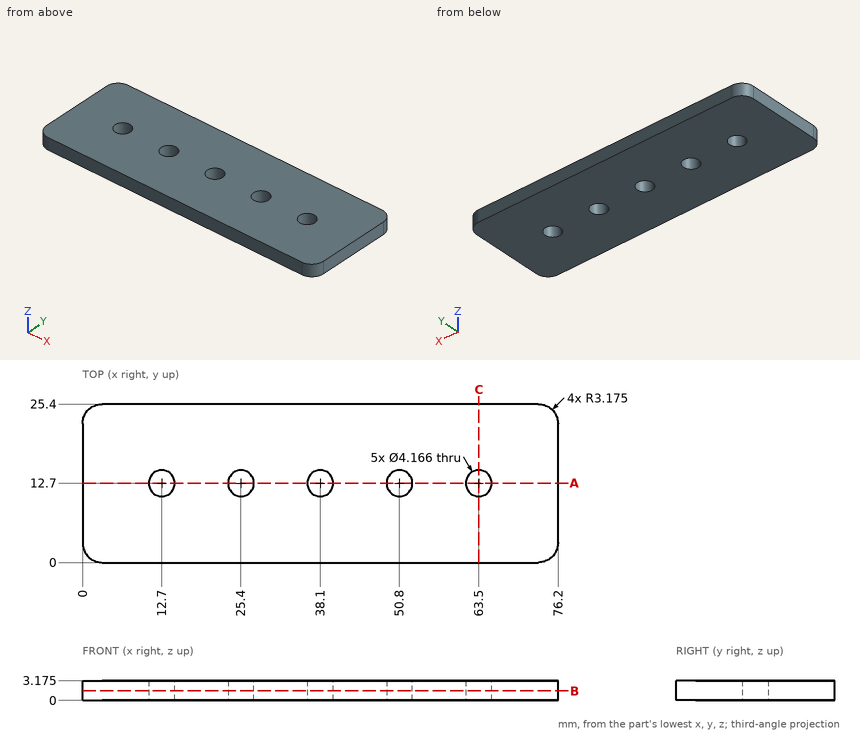
Job drawing, mm, ordinate dimensions from the low corner. One solid piece. Give positions to 0.01 mm unless a question says otherwise; leave off trailing zeros. Write each loop counter-clockwise with the first axis right and the second up, starting at its lowest first coordinate (ties: lowest second). Pieces come first, ordered by that corner, then holes. Notation, with made-up numbers: M 24,31.5 L 66,31.5 A15 ccw 66,55.5 Z; hole C 2.25,-5.5 d7. An arc over 180 degrees is marked long. Put each result on its own line as item: value. Start each with the question number.
(1) Probe L1, parallel to X at y = 11.5, z = 1.9; L2, parallel to Y at x = 25.4, z = 1.15; L3, parallel to Y at x = 12, z = 0.4. List the from-to ranges inside material, lowest first.
(2) Band-saw the part on A-A, the plane y = 12.7. Write the cut outline in (x, z) (1 decimal), and give its area (3 significant figures).
(3) Band-saw the part on C-C, the plane x = 63.5. Write the cut outline in (y, z) (1 decimal).
(4) Band-saw the part on B-B, the plane z = 1.5. Give the number of separate pieces and of enclosed holes in the cut face, and give its area (3 significant figures).
Response values:
1. L1: x = 0 to 11, 14.4 to 23.7, 27.1 to 36.4, 39.8 to 49.1, 52.5 to 61.8, 65.2 to 76.2
1. L2: y = 0 to 10.62, 14.78 to 25.4
1. L3: y = 0 to 10.74, 14.66 to 25.4
2. outline: M 0,0 L 10.6,0 L 10.6,3.2 L 0,3.2 Z; M 14.8,0 L 23.3,0 L 23.3,3.2 L 14.8,3.2 Z; M 27.5,0 L 36,0 L 36,3.2 L 27.5,3.2 Z; M 40.2,0 L 48.7,0 L 48.7,3.2 L 40.2,3.2 Z; M 52.9,0 L 61.4,0 L 61.4,3.2 L 52.9,3.2 Z; M 65.6,0 L 76.2,0 L 76.2,3.2 L 65.6,3.2 Z
2. area: 176 mm2
3. outline: M 0,0 L 10.6,0 L 10.6,3.2 L 0,3.2 Z; M 14.8,0 L 25.4,0 L 25.4,3.2 L 14.8,3.2 Z
4. separate pieces: 1
4. enclosed holes: 5
4. area: 1,860 mm2
